from build123d import *

# Parameters (mm, degrees)
SKETCH_1_R          = 7.5
EXTRUDE_1_DEPTH     = 5
SKETCH_2_R          = 5
CUT_EXTRUDE_1_DEPTH = 2
SKETCH_3_R          = 3.4
CUT_EXTRUDE_2_DEPTH = 12.022703843
SKETCH_4_W          = 6
SKETCH_4_H          = 11
EXTRUDE_2_DEPTH     = 5
FILLET_1_R          = 2
SKETCH_8_R          = 1
CUT_EXTRUDE_4_DEPTH = 15.221462653
SKETCH_9_W          = 7
SKETCH_9_H          = 7.5
EXTRUDE_3_DEPTH     = 5
FILLET_2_R          = 2


with BuildPart() as part:
    # 草图1 → 凸台-拉伸1 (new body)
    with BuildSketch(Plane(origin=(0, 0, 0), x_dir=(0, 0, -1), z_dir=(1, 0, 0))):
        Circle(SKETCH_1_R)
    extrude(amount=EXTRUDE_1_DEPTH)

    # 草图2 → 切除-拉伸1 (cut)
    with BuildSketch(Plane.ZY):
        Circle(SKETCH_2_R)
    extrude(amount=-CUT_EXTRUDE_1_DEPTH, mode=Mode.SUBTRACT)

    # 草图3 → 切除-拉伸2 (cut, through all)
    with BuildSketch(Plane.ZY.offset(-2)):
        Circle(SKETCH_3_R)
    extrude(amount=-CUT_EXTRUDE_2_DEPTH, mode=Mode.SUBTRACT)

    # 草图4 → 凸台-拉伸2 (add)
    with BuildSketch(Plane.ZY):
        with Locations((8, 0)):
            Rectangle(SKETCH_4_W, SKETCH_4_H)
        with Locations((-8, 0)):
            Rectangle(SKETCH_4_W, SKETCH_4_H)
    extrude(amount=-EXTRUDE_2_DEPTH)

    # 草图6 → 切除-旋转1 (revolve, cut)
    with BuildSketch(Plane.ZY):
        with BuildLine():
            Line((8, 2.65), (8, -2.65))
            ThreePointArc((8, -2.65), (10.65, 0), (8, 2.65))
        make_face()
    revolve(axis=Axis((0, 2.65, 8), (0, -1, 0)), mode=Mode.SUBTRACT)

    # 草图7 → 切除-旋转2 (revolve, cut)
    with BuildSketch(Plane.ZY):
        with BuildLine():
            Line((-8, 2.65), (-8, -2.65))
            ThreePointArc((-8, -2.65), (-5.35, 0), (-8, 2.65))
        make_face()
    revolve(axis=Axis((0, 2.65, -8), (0, -1, 0)), mode=Mode.SUBTRACT)

    # 圆角1
    fillet_1_edges = [part.edges().sort_by_distance(p)[0] for p in [
        (2.5, -5.5, 11),
        (2.5, 5.5, 11),
        (2.5, 5.5, -11),
        (2.5, -5.5, -11),
    ]]
    fillet(fillet_1_edges, radius=FILLET_1_R)

    # 草图8 → 切除-拉伸4 (cut, through all)
    with BuildSketch(Plane.ZY):
        with Locations((8.5, -3.7)):
            Circle(SKETCH_8_R)
        with Locations(Location((8.5, 3.7, 0), (0, 0, 180))):
            Circle(SKETCH_8_R)
        with Locations(Location((-8.5, -3.7, 0), (0, 0, 180))):
            Circle(SKETCH_8_R)
        with Locations((-8.5, 3.7)):
            Circle(SKETCH_8_R)
    extrude(amount=-CUT_EXTRUDE_4_DEPTH, mode=Mode.SUBTRACT)

    # 草图9 → 凸台-拉伸3 (add)
    with BuildSketch(Plane(origin=(5, 0, 0), x_dir=(0, 0, -1), z_dir=(1, 0, 0))):
        with Locations((0, -9.25)):
            Rectangle(SKETCH_9_W, SKETCH_9_H)
    extrude(amount=-EXTRUDE_3_DEPTH)

    # 草图10 → 切除-旋转3 (revolve, cut)
    with BuildSketch(Plane.ZY):
        with BuildLine():
            Line((0, -7.35), (0, -12.65))
            ThreePointArc((0, -12.65), (-2.65, -10), (0, -7.35))
        make_face()
    revolve(axis=Axis((0, -7.35, 0), (0, -1, 0)), mode=Mode.SUBTRACT)

    # 圆角2
    fillet_2_edges = [part.edges().sort_by_distance(p)[0] for p in [
        (2.5, -13, 3.5),
        (2.5, -13, -3.5),
    ]]
    fillet(fillet_2_edges, radius=FILLET_2_R)


solid = part.part
Model file for the job. Use its own axes, mm. A direction names the side the tool comes from. Coordinates: 2 decimals unless noted, no trailing zeros. Order: outer loops, then holes, each group sorted by start corner. A loop starts at its lowest first (then second) coordinate and runs counter-clockwise, first axis right, second up. Notation, with made-up numbers: M -19.5,-35 L 39.5,-35 A12 cw 39.5,-18 Z; hole C -36.5,80.25 d4. An arc over 180 degrees is marked long. Return JSON: item names as keys, results as strings.
1. Saw through at C-C (x = 3.45). Give the cut face in (y, z).
Ans:
{"outline": "M -13,-1.5 A2 ccw -11,-3.5 L -6.63,-3.5 A7.5 ccw -5.5,-5.1 L -5.5,-9 A2 ccw -3.5,-11 L 3.5,-11 A2 ccw 5.5,-9 L 5.5,-5.1 A7.5 ccw 5.5,5.1 L 5.5,9 A2 ccw 3.5,11 L -3.5,11 A2 ccw -5.5,9 L -5.5,5.1 A7.5 ccw -6.63,3.5 L -11,3.5 A2 ccw -13,1.5 Z; hole C -3.7,-8.5 d2; hole C -3.7,8.5 d2; hole C 0,0 d6.8; hole C 3.7,-8.5 d2; hole C 3.7,8.5 d2"}
2. Saw through at B-B (y = 0). Give the cut face in (x, z), and give its area (3 significant figures).
Ans:
{"outline": "M 0,-11 L 5,-11 L 5,-3.4 L 2,-3.4 L 2,-5 L 0,-5 L 0,-5.35 A2.65 cw 0,-10.65 Z; M 0,5 L 2,5 L 2,3.4 L 5,3.4 L 5,11 L 0,11 L 0,10.65 A2.65 cw 0,5.35 Z", "area": "47.5 mm^2"}
3. Tool access for faces 1 (the face through (2, -5.5, 7)), 2 (the face through (3, -9, -3.5)), 3 (the face through (2, 5.5, 7)): list every direction of +Z, -Z, +X, -X, +Y, -Y with a clear straight run to the whole face (end or side of a thin tool).
Ans:
{"face 1": "+Z, +X, -X, -Y", "face 2": "-Z, +X, -X, -Y", "face 3": "+Z, +X, -X, +Y"}
4. Drill centre lines: probe 1 along Y at (x, z) = (3.25, -8.5); probe 2 along Y at (x, z) = (1.6, 0.25); probe 3 along Z at (x, y) = (1.6, -1). Where is each one in solid material? Low to high.
Ans:
{"probe 1": "-5.5 to -4.7, -2.7 to 2.7, 4.7 to 5.5", "probe 2": "-13 to -12.1, -7.9 to -4.99, 4.99 to 7.5", "probe 3": "-11 to -9.86, -6.14 to -4.9, 4.9 to 6.14, 9.86 to 11"}
5. Flat gauge pins, fed straight in: pin 1 (1 mm diameter, centred on x = 2.5, y = -11, fed in from +Z); pin 2 (2 mm diameter, centred on x = 1.5, y = -8, fed in from -Z); pin 3 (1.2 mm diameter, centred on x = 2, z = 8, fed in from -Y). Where does each tip first touch, or does it go through?
Ans:
{"pin 1": "z = 3.5", "pin 2": "z = -3.5", "pin 3": "y = -5.5"}
6. Pull direction Y, two halves, no side cores. Call faces 4 (the face through (2.54, -4.9, -10.43)), 5 (the face through (0.99, -4.88, -1.08)), 6 (the face through (0, -5, 3)): +Y half, -Y half, draft (parallel to the pull), parting line (faces both ways), or undercut.
Ans:
{"face 4": "-Y half", "face 5": "undercut", "face 6": "draft"}
7. Saw through at A-A (z = 0). Give the cut face in (x, y).
Ans:
{"outline": "M 0,-13 L 5,-13 L 5,-3.4 L 2,-3.4 L 2,-5 L 0,-5 L 0,-7.35 A2.65 cw 0,-12.65 Z; M 0,5 L 2,5 L 2,3.4 L 5,3.4 L 5,7.5 L 0,7.5 Z"}
8. Saw through at D-D (z = 5.75). Give the cut face in (x, y).
Ans:
{"outline": "M 0,-5.5 L 5,-5.5 L 5,5.5 L 0,5.5 L 0,1.4 A1.4 cw 0,-1.4 Z"}
